from build123d import *

# Parameters (mm, degrees)
SKETCH1_W          = 3.937
SKETCH1_H          = 38.608
HOLE1_D            = 3.96748
HOLE1_DEPTH        = 11.684
HOLE1_CSINK_D      = 4.826
HOLE1_CSINK_ANGLE  = 90
SKETCH4_W          = 12.7
SKETCH4_H          = 31.496
SKETCH4_W_2        = 6.35
SKETCH4_H_2        = 15.748
CUT_EXTRUDE1_DEPTH = 3.302


with BuildPart() as part:
    # Sketch1 → Revolve1 (revolve)
    with BuildSketch(Plane.XY):
        with Locations((1.9685, 19.304)):
            Rectangle(SKETCH1_W, SKETCH1_H)
    revolve(axis=Axis((0, 0, 0), (0, 1, 0)))

    # Hole1
    with Locations(Plane(origin=(0, 38.608, 0), x_dir=(1, 0, 0), z_dir=(0, 1, 0))):
        with Locations((0, 0)):
            CounterSinkHole(HOLE1_D / 2, HOLE1_CSINK_D / 2, depth=HOLE1_DEPTH, counter_sink_angle=HOLE1_CSINK_ANGLE)

    # Sketch4 → Cut-Extrude1 (cut)
    with BuildSketch(Plane(origin=(0, 38.608, 0), x_dir=(1, 0, 0), z_dir=(0, 1, 0))):
        Rectangle(SKETCH4_W, SKETCH4_H)
        Rectangle(SKETCH4_W_2, SKETCH4_H_2, mode=Mode.SUBTRACT)
    extrude(amount=-CUT_EXTRUDE1_DEPTH, mode=Mode.SUBTRACT)


solid = part.part
Could you check a few things on this model? Use its own coordinates, in mm. A direction names the side the tool comes from. Give positions to 0.01 mm unless a question says otherwise; leave off trailing zeros. Write each loop counter-clockwise with the first axis right and the second up, starting at its lowest first coordinate (ties: lowest second). Pieces come first, ordered by that corner, then holes. Notation, with made-up numbers: (-19, -23) -> (19, -23) arc R28 cw to (19, 15) -> close; hole circle Ø2 at (-28.5, -12). An arc over 180 degrees is marked (long way). Write each question's results on one line, items separated by ' | '. Start each with the question number.
Q1. Suppose I cut it at B-B, the plane z = 0. List the corners of the cut face in (x, y) for me (3 decimals), and give its area (3 significant figures).
Q2. I'm going to push flat-ended pins straight in: pin 1 Ø1.2 at (x, z) = (0, -1) entering from +Y; pin 2 Ø3 at (y, z) = (28, -2.5) entering from -X; pin 3 Ø1.5 at (x, y) = (1.5, 28.5) entering from +Z. Where does each tip first touch, or does it pass through?
Q3. Suppose I cut it at A-A, the plane x = 0. List the corners of the cut face in (y, z) for me, and give its area (3 significant figures).
Q4. I need wall thicknesses on probe 1 along Z at (x, y) = (0, 29.5); probe 2 along Y at (x, z) = (0.25, -1.5); probe 3 along X at (y, z) = (33.5, 1.25). Which ranges of each line are inside material? Lowest first, please.
Q5. Suppose I cut it at C-C, the plane y = 32.5. List the corners of the cut face in (x, z) for me.
Q6. Which directions (+Z, -Z, +X, -X, +Y, -Y) give clear straight access to the entire face, cutting with the end or side of a thin tool? Please do faces 4 (the face through (0.258, 32.473, -1.967)), 5 (the face through (0, 0, 0)), 6 (the face through (-3.175, 37, 0)).
Q7. Suppose I cut it at D-D, the plane y = 9. List the corners of the cut face in (x, z) for me.
Q8. We'd pull the mould along X, two halves only. Please class faces 1 (the face through (-3.933, 19.574, -0.173)), 2 (the face through (0, 26.924, 0)), 3 (the face through (3.175, 37, 0)): +X half, -X half, draft (parallel to the pull), parting line (faces both ways), or undercut.
Outcome:
1) outline: (-3.937, 0) -> (3.937, 0) -> (3.937, 35.306) -> (3.175, 35.306) -> (3.175, 38.608) -> (2.413, 38.608) -> (1.984, 38.179) -> (1.984, 26.924) -> (-1.984, 26.924) -> (-1.984, 38.179) -> (-2.413, 38.608) -> (-3.175, 38.608) -> (-3.175, 35.306) -> (-3.937, 35.306) -> close | area: 252 mm2
2) pin 1: y = 26.92 | pin 2: x = -3.81 | pin 3: z = 3.86
3) outline: (0, -3.94) -> (38.61, -3.94) -> (38.61, -2.41) -> (38.18, -1.98) -> (26.92, -1.98) -> (26.92, 1.98) -> (38.18, 1.98) -> (38.61, 2.41) -> (38.61, 3.94) -> (0, 3.94) -> close | area: 257 mm2
4) probe 1: -3.94 to -1.98, 1.98 to 3.94 | probe 2: 0 to 26.92 | probe 3: -3.73 to -1.54, 1.54 to 3.73
5) outline: circle Ø7.87 at (0, 0); hole circle Ø3.97 at (0, 0)
6) face 4: +Y | face 5: +Z, -Z, +X, -X, -Y | face 6: +Z, -Z, -X, +Y
7) outline: circle Ø7.87 at (0, 0)
8) face 1: parting line | face 2: undercut | face 3: +X half
